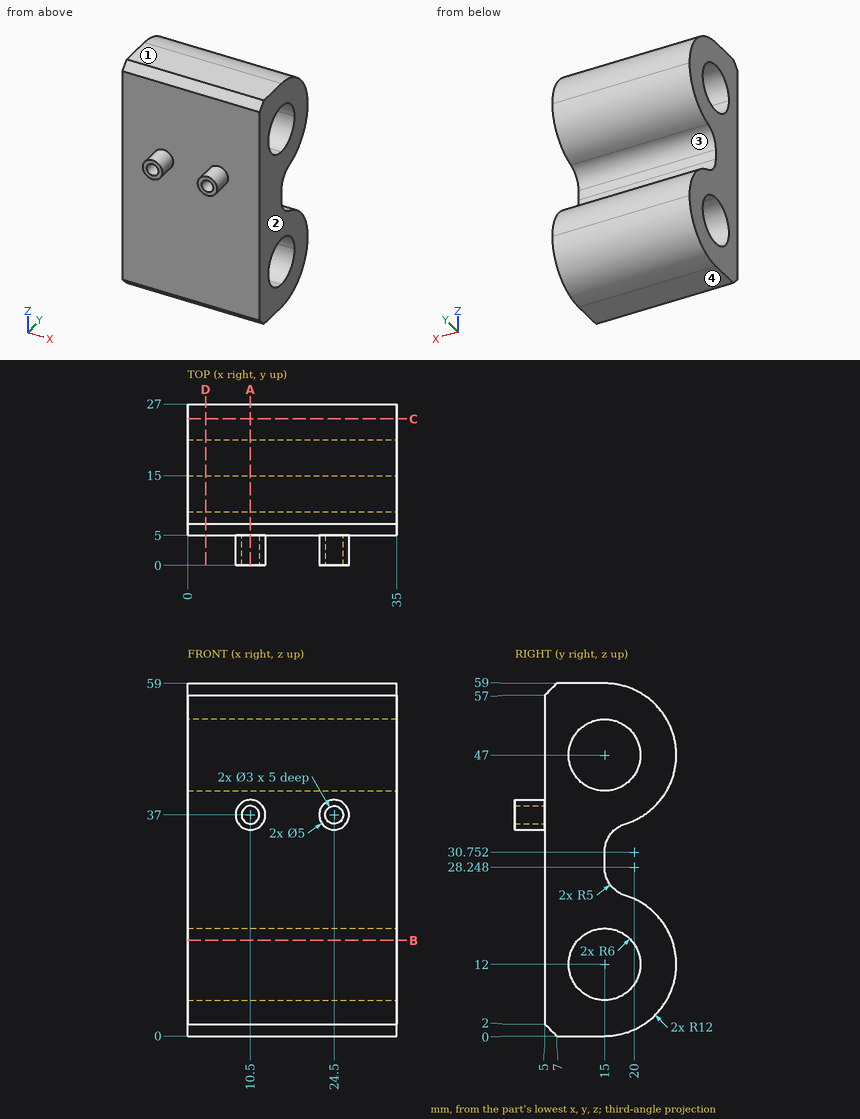
Print and shaded views of the part. All mm, measured from the part's lowest x, y and z. Give positions to 0.01 mm unless a question says otherwise; leave off trailing zeros. Order: outer loops, then holes, each group sorted by start corner. A loop starts at its lowest first (then second) coordinate and runs counter-clockwise, first axis right, second up. Notation, with made-up numbers: (4.25, 3) - (9.25, 3) arc R18 ccw to (9.25, 17) - close; hole circle Ø8 at (11.25, 75). An arc over 180 degrees is marked (long way). Use a Markdown table: item, result.
1) Two-plate mould, pull along Z, no slides. Class the marked faces 1, 2, 3 and 4: +Z half, -Z half, draft (parallel to the pull), parting line (faces both ways), or undercut.
Checked values:
| item | result |
|---|---|
| face 1 | +Z half |
| face 2 | draft |
| face 3 | undercut |
| face 4 | -Z half |
2) Probe L1, parallel to Z at x = 10.5, y = 12.5; L2, parallel to Z at x = 10.5, y = 2; L3, parallel to Z at x = 33, y = 13.5. List the from-to ranges inside material, lowest first. Write a range as from..to.
Checked values:
| item | result |
|---|---|
| L1 | 0..6.55, 17.45..41.55, 52.45..59 |
| L2 | 34.5..35.5, 38.5..39.5 |
| L3 | 0..6.19, 17.81..41.19, 52.81..59 |
3) Flat gauge pins, fed straight in: P1, Ø12, axis at x = 19.5, z = 40.5, coming from the +Y side; P2, Ø3.5, axis at x = 24.5, z = 37, coming from the +Y side; P3, Ø4, axis at x = 5.5, z = 7.5, coming from the -Y side. Where does each tip first touch, or does it go through?
Checked values:
| item | result |
|---|---|
| P1 | y = 26.99 |
| P2 | y = 23.71 |
| P3 | y = 5 |
4) Saw through at C-C on y = 24.5. List the corners of the cut face in (x, z).
Checked values:
| item | result |
|---|---|
| outline | (0, 4.67) - (35, 4.67) - (35, 19.33) - (0, 19.33) - close; (0, 39.67) - (35, 39.67) - (35, 54.33) - (0, 54.33) - close |
5) Saw through at B-B on z = 16. List the corners of the cut face in (x, y).
Checked values:
| item | result |
|---|---|
| outline | (0, 5) - (35, 5) - (35, 10.53) - (0, 10.53) - close; (0, 19.47) - (35, 19.47) - (35, 26.31) - (0, 26.31) - close |
6) Saw through at A-A on x = 10.5. List the corners of the cut face in (y, z).
Checked values:
| item | result |
|---|---|
| outline | (0, 34.5) - (5, 34.5) - (5, 2) - (7, 0) - (15, 0) arc R12 ccw to (18.53, 23.47) arc R5 cw to (15, 28.25) - (15, 30.75) arc R5 cw to (18.53, 35.53) arc R12 ccw to (15, 59) - (7, 59) - (5, 57) - (5, 39.5) - (0, 39.5) - (0, 38.5) - (5, 38.5) - (5, 35.5) - (0, 35.5) - close; hole circle Ø12 at (15, 12); hole circle Ø12 at (15, 47) |
7) Saw through at D-D on x = 3. List the corners of the cut face in (y, z), plus the area to 3 significant figures.
Checked values:
| item | result |
|---|---|
| outline | (5, 2) - (7, 0) - (15, 0) arc R12 ccw to (18.53, 23.47) arc R5 cw to (15, 28.25) - (15, 30.75) arc R5 cw to (18.53, 35.53) arc R12 ccw to (15, 59) - (7, 59) - (5, 57) - close; hole circle Ø12 at (15, 12); hole circle Ø12 at (15, 47) |
| area | 819 mm² |
